The listing builds one solid part. Answer for the finished solid, in the listing's coordinates (mm). A direction names the side the tool comes from. Coordinates: 2 decimals unless noted, no trailing zeros. Loops run counter-clockwise (first coordinate to the right, second up) from the corner with the lowest first, then second, coordinate; pieces in that order, holes last. Notation, with made-up numbers: (-12.75, 84.25) - (33.25, 84.25) arc R27 cw to (33.25, 113.25) - close; hole circle Ø11 at (14, -26.5). An arc over 180 degrees is marked (long way). Write each question's results on one line, items separated by ' | '. Start each with the question number.
(1) Find section C-C on x = 17.5. Determine the outline of the cut face in (y, z).
(2) Find section A-A on y = -8. Determine the outline of the cut face in (x, z).
(3) Find section B-B on z = -11.75. Determine the outline of the cut face in (x, y), then the cut area to 3 significant figures.
(4) For faces 1 (the flat face through (9.5, 0, -9.9)), 2 (the flat face through (10, -5, -17)), determine the directions among +Z, -Z, +X, -X, +Y, -Y from which every point of the face is accessible in a straight line to the end or side of a thin tool.
(5) Consider line 1 (X direction, y = -5.75, z = -12.5); line 2 (Z direction, x = 16, y = -2.5). Determine where each line is inside the solid, lowest interval first. Write a range as from..to.
(6) Given pin 1 Ø5 at (y, z) = (-5.5, -13.5) entering from +X, flat-ended and moving along its own axis, determine where the tip first touches the part or whether it passes through.
from build123d import *

# Parameters (mm, degrees)
SKETCH1_W           = 15
SKETCH1_H           = 10
SKETCH1_W_2         = 10
SKETCH1_H_2         = 15
BOSS_EXTRUDE2_DEPTH = 10


with BuildPart() as part:
    # Sketch1 → Boss-Extrude2 (new body)
    with BuildSketch(Plane(origin=(0, 0, 0), x_dir=(1, 0, 0), z_dir=(0, 1, 0))):
        with Locations((17.5, 5)):
            Rectangle(SKETCH1_W, SKETCH1_H)
        with Locations((5, 5)):
            Rectangle(SKETCH1_W_2, SKETCH1_H)
        with Locations((5, 17.5)):
            Rectangle(SKETCH1_W_2, SKETCH1_H_2)
    extrude(amount=-BOSS_EXTRUDE2_DEPTH)


solid = part.part
Values:
1) outline: (-10, -10) - (0, -10) - (0, 0) - (-10, 0) - close
2) outline: (0, -25) - (10, -25) - (10, -10) - (25, -10) - (25, 0) - (0, 0) - close
3) outline: (0, -10) - (10, -10) - (10, 0) - (0, 0) - close | area: 100 mm²
4) face 1: +Z, -Z, +X, -X, +Y | face 2: -Z, +X, +Y, -Y
5) line 1: x = 0..10 | line 2: z = -10..0
6) pin 1: stops at x = 10
